Could you check a few things on this model? Use its own coordinates, in mm. Face numbers are marked on the shaded views. Coordinates: 2 decimals unless noted, no trailing zeros. Order: outer loops, then holes, each group sorted by start corner. A loop starts at its lowest first (then second) coordinate and runs counter-clockwise, first axis right, second up. Notation, with made-up numbers: (60.5, -0.5) - (111.5, -0.5) arc R24 ccw to (111.5, 11.5) - close; hole circle Ø1 at (-6, 8). An arc over 180 degrees is marked (long way). Answer as a JSON object with one key per item and string values. Group by question number.
(1) We'd pull the mould along Z, two halves only. Please class the marked faces 1 and 2: pulls with the +Z half, pulls with the -Z half, needs draft (parallel to the pull), parting line crosses it, or undercut.
(2) Please list where these lines run through material, in increasing order: probe 1 along Y at (x, z) = (0, 1.2); probe 2 along X at (y, z) = (15.5, 0.45); probe 3 along X at (y, z) = (-16, 1).
(3) Imagine slicing it at D-D, the plane y = -15. Write out the boundary of the cut face in (x, z), and give its area (3 significant figures).
(4) Imagine slicing it at C-C, the plane y = 8.5. Write out the boundary of the cut face in (x, z).
(5) Imagine slicing it at B-B, the plane z = 1.25. Write out the boundary of the cut face in (x, y).
(6) Will this pin go through, and if not, where does the flat tip stop? P1, Ø12, axis at x = -2.5, y = -10.5, coming from the -Z side.
(7) Imagine slicing it at A-A, the plane x = 0. Write out the boundary of the cut face in (y, z), and give its area (3 significant figures).
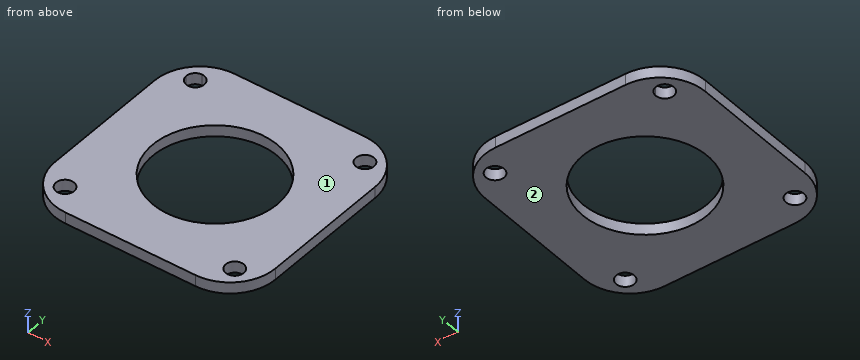
from build123d import *

# Parameters (mm, degrees)
SKETCH_1_R          = 1.6
SKETCH_1_R_2        = 5.5
EXTRUDE_2_DEPTH     = 2
FILLET_6_R          = 8
FILLET_7_R          = 8
FILLET_8_R          = 8
FILLET_9_R          = 8
SKETCH_2_R          = 11
CUT_EXTRUDE_1_DEPTH = 10


with BuildPart() as part:
    # 草图1 → 凸台-拉伸2 (new body)
    # profile 1 of 2: a face of its own
    with BuildSketch(Plane.XY):
        with BuildLine():
            Line((-16.6, 15), (-19.5, 15))
            Line((-19.5, 15), (-19.5, -19.5))
            Line((-19.5, -19.5), (19.5, -19.5))
            Line((19.5, -19.5), (19.5, 19.5))
            Line((19.5, 19.5), (-15, 19.5))
            Line((-15, 19.5), (-15, 16.6))
            ThreePointArc((-15, 16.6), (-13.86862915, 16.13137085), (-13.4, 15))
            ThreePointArc((-13.4, 15), (-15, 13.4), (-16.6, 15))
        make_face()
        with Locations((-15, -15)):
            Circle(SKETCH_1_R, mode=Mode.SUBTRACT)
        with Locations((15, -15)):
            Circle(SKETCH_1_R, mode=Mode.SUBTRACT)
        Circle(SKETCH_1_R_2, mode=Mode.SUBTRACT)
        with Locations((15, 15)):
            Circle(SKETCH_1_R, mode=Mode.SUBTRACT)
    # profile 2 of 2: a face of its own
    with BuildSketch(Plane.XY):
        with BuildLine():
            Line((-19.5, 19.5), (-19.5, 15))
            Line((-19.5, 15), (-16.6, 15))
            ThreePointArc((-16.6, 15), (-16.13137085, 16.13137085), (-15, 16.6))
            Line((-15, 16.6), (-15, 19.5))
            Line((-15, 19.5), (-19.5, 19.5))
        make_face()
    extrude(amount=EXTRUDE_2_DEPTH)

    # 圆角6
    fillet_6_edges = [part.edges().sort_by_distance(p)[0] for p in [
        (-19.5, 19.5, 1),
    ]]
    fillet(fillet_6_edges, radius=FILLET_6_R)

    # 圆角7
    fillet_7_edges = [part.edges().sort_by_distance(p)[0] for p in [
        (19.5, 19.5, 1),
    ]]
    fillet(fillet_7_edges, radius=FILLET_7_R)

    # 圆角8
    fillet_8_edges = [part.edges().sort_by_distance(p)[0] for p in [
        (-19.5, -19.5, 1),
    ]]
    fillet(fillet_8_edges, radius=FILLET_8_R)

    # 圆角9
    fillet_9_edges = [part.edges().sort_by_distance(p)[0] for p in [
        (19.5, -19.5, 1),
    ]]
    fillet(fillet_9_edges, radius=FILLET_9_R)

    # 草图2 → 切除-拉伸1 (cut)
    with BuildSketch(Plane.XY.offset(2)):
        Circle(SKETCH_2_R)
    extrude(amount=-CUT_EXTRUDE_1_DEPTH, mode=Mode.SUBTRACT)


solid = part.part
Result set:
{
 "1": {"face 1": "pulls with the +Z half", "face 2": "pulls with the -Z half"},
 "2": {"probe 1": "y = -19.5 to -11, 11 to 19.5", "probe 2": "x = -18.43 to -16.52, -13.48 to 13.48, 16.52 to 18.43", "probe 3": "x = -18.11 to -16.25, -13.75 to 13.75, 16.25 to 18.11"},
 "3": {"outline": "(-18.69, 0) - (-16.6, 0) - (-16.6, 2) - (-18.69, 2) - close; (-13.4, 0) - (13.4, 0) - (13.4, 2) - (-13.4, 2) - close; (16.6, 0) - (18.69, 0) - (18.69, 2) - (16.6, 2) - close", "area": "62.0 mm^2"},
 "4": {"outline": "(-19.5, 0) - (-6.98, 0) - (-6.98, 2) - (-19.5, 2) - close; (6.98, 0) - (19.5, 0) - (19.5, 2) - (6.98, 2) - close"},
 "5": {"outline": "(-19.5, -11.5) arc R8 ccw to (-11.5, -19.5) - (11.5, -19.5) arc R8 ccw to (19.5, -11.5) - (19.5, 11.5) arc R8 ccw to (11.5, 19.5) - (-11.5, 19.5) arc R8 ccw to (-19.5, 11.5) - close; hole circle Ø3.2 at (-15, -15); hole circle Ø3.2 at (-15, 15); hole circle Ø22 at (0, 0); hole circle Ø3.2 at (15, -15); hole circle Ø3.2 at (15, 15)"},
 "6": {"P1": "stops at z = 0"},
 "7": {"outline": "(-19.5, 0) - (-11, 0) - (-11, 2) - (-19.5, 2) - close; (11, 0) - (19.5, 0) - (19.5, 2) - (11, 2) - close", "area": "34.0 mm^2"}
}
